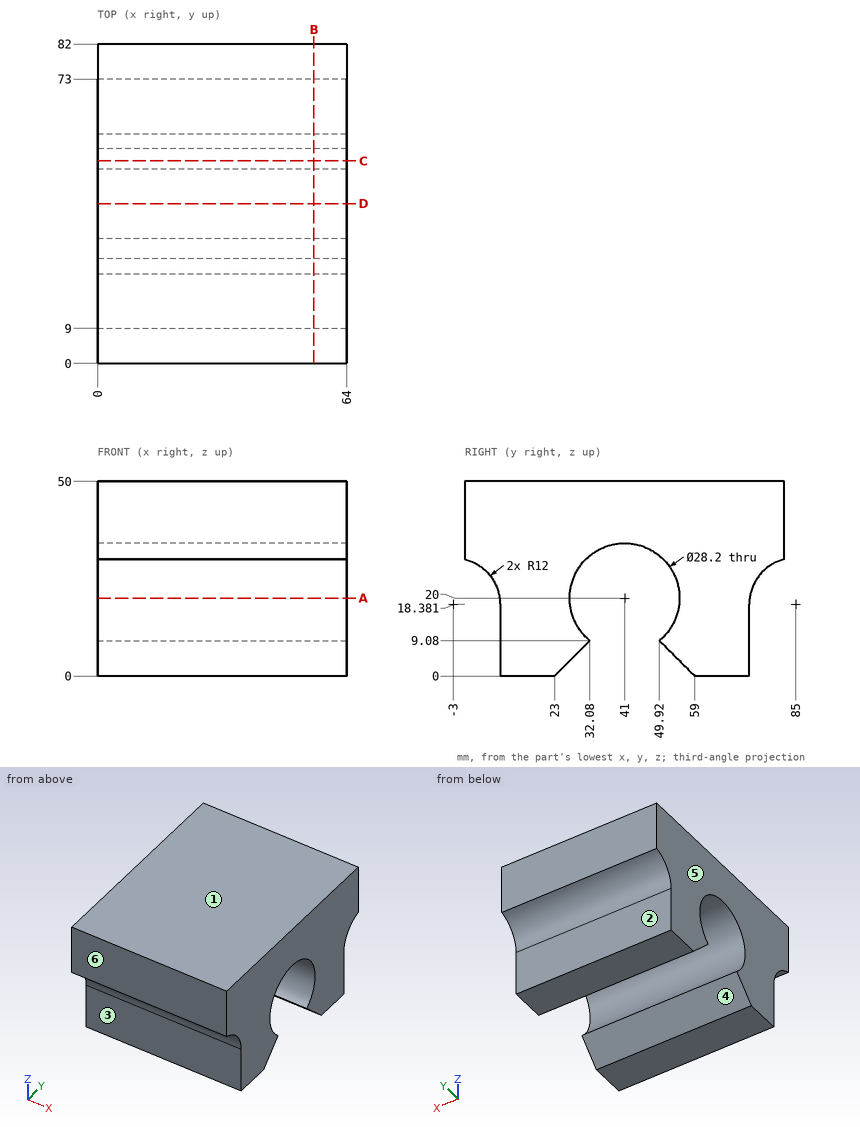
Could you check a few things on this drawing? It's one solid part, dimensions in mm from its lowest x, y, z. A direction names the side the tool comes from. Coordinates: 2 decimals unless noted, no trailing zeros. Order: outer loops, then holes, each group sorted by start corner. A loop starts at its lowest first (then second) coordinate and runs counter-clockwise, first axis right, second up. Notation, with made-up numbers: M 23.25,76.5 L 45.25,76.5 A16 ccw 45.25,83.5 Z; hole C 46,85 d10. An arc over 180 degrees is marked long. Use a Markdown table: item, result. Add a question column.
Q1. Which directions (+Z, -Z, +X, -X, +Y, -Y) give clear straight access to the entire face, cutting with the end or side of a thin tool? Please do the marked faces 1, 2 and 3.
Q2. I want a section at B-B on x = 55.5. List the corners of the cut face in (y, z) for me.
Q3. I want a section at D-D on y = 41. List the corners of the cut face in (x, z) for me, then the cut area to 3 significant figures.
Q4. I want a section at A-A on z = 20. List the corners of the cut face in (x, y) for me, then the cut area to 3 significant figures.
Q5. I'm going to push flat-ended pins straight in: pin 1 (10 mm diameter, centred on x = 23, z = 14, fed in from -Y); pin 2 (1.5 mm diameter, centred on x = 50.5, z = 26.5, fed in from +Y); pin 3 (4 mm diameter, centred on y = 67, z = 22, fed in from -X); pin 4 (10 mm diameter, centred on x = 41, z = 19.5, fed in from -Y). Where does each tip first touch, or does it pass through?
Q6. If I drill on L1, parallel to Y at x = 15, z = 20; L2, parallel to Y at x = 48.5, z = 5; L3, parallel to Z at x = 45, y = 75.5, over which ranges is the centre line in solid material (lowest first)?
Q7. We'd pull the mould along Y, two halves only. Please class the marked faces 4, 5 and 6: pulls with the +Y half, pulls with the -Y half, needs draft (parallel to the pull), parting line crosses it, or undercut.
Q8. I want a section at C-C on y = 52. List the corners of the cut face in (x, z) for me, then the cut area to 3 significant figures.
Checked values:
| question | item | result |
|---|---|---|
| 1 | face 1 | +Z, +X, -X, +Y, -Y |
| 1 | face 2 | -Z, +X, -X, +Y |
| 1 | face 3 | -Z, +X, -X, -Y |
| 2 | outline | M 0,30 A12 cw 9,18.38 L 9,0 L 23,0 L 32.08,9.08 A14.1 cw long 49.92,9.08 L 59,0 L 73,0 L 73,18.38 A12 cw 82,30 L 82,50 L 0,50 Z |
| 3 | outline | M 0,34.1 L 64,34.1 L 64,50 L 0,50 Z |
| 3 | area | 1,020 mm² |
| 4 | outline | M 0,8.89 L 64,8.89 L 64,26.9 L 0,26.9 Z; M 0,55.1 L 64,55.1 L 64,73.11 L 0,73.11 Z |
| 4 | area | 2,310 mm² |
| 5 | pin 1 | y = 8.98 |
| 5 | pin 2 | y = 76.92 |
| 5 | pin 3 | x = 0 |
| 5 | pin 4 | y = 7.32 |
| 6 | L1 | 8.89 to 26.9, 55.1 to 73.11 |
| 6 | L2 | 9 to 28, 54 to 73 |
| 6 | L3 | 25.71 to 50 |
| 7 | face 4 | undercut |
| 7 | face 5 | needs draft |
| 7 | face 6 | pulls with the -Y half |
| 8 | outline | M 0,7 L 64,7 L 64,11.18 L 0,11.18 Z; M 0,28.82 L 64,28.82 L 64,50 L 0,50 Z |
| 8 | area | 1,620 mm² |
